from build123d import *

# Parameters (mm, degrees)
SKETCH_1_R      = 23
SKETCH_1_R_2    = 1.75
SKETCH_1_R_3    = 5
EXTRUDE_1_DEPTH = 3
SKETCH_1_3_R    = 5
EXTRUDE_2_DEPTH = 32.75
SKETCH_2_R      = 25
SKETCH_2_R_2    = 1.75
EXTRUDE_3_DEPTH = 3


with BuildPart() as part:
    # 草图1 → 凸台-拉伸1 (new body)
    with BuildSketch(Plane(origin=(0, 0, 0), x_dir=(1, 0, 0), z_dir=(0, 1, 0))):
        with Locations(Location((7.5, 0, 0), (0, 0, 270))):
            Circle(SKETCH_1_R)
        with Locations(Location((27.5, 0, 0), (0, 0, 270))):
            Circle(SKETCH_1_R_2, mode=Mode.SUBTRACT)
        with Locations(Location((-12.5, 0, 0), (0, 0, 270))):
            Circle(SKETCH_1_R_2, mode=Mode.SUBTRACT)
        with Locations(Location((0, 0, 0), (0, 0, 270))):
            Circle(SKETCH_1_R_3, mode=Mode.SUBTRACT)
        with Locations(Location((15, 0, 0), (0, 0, 270))):
            Circle(SKETCH_1_R_3, mode=Mode.SUBTRACT)
    extrude(amount=EXTRUDE_1_DEPTH)

    # 草图1<3> → 凸台-拉伸2 (add)
    with BuildSketch(Plane(origin=(0, 0, 0), x_dir=(1, 0, 0), z_dir=(0, 1, 0))):
        with Locations(Location((0, 0, 0), (0, 0, 270))):
            Circle(SKETCH_1_3_R)
        with Locations(Location((15, 0, 0), (0, 0, 270))):
            Circle(SKETCH_1_3_R)
    extrude(amount=EXTRUDE_2_DEPTH)

    # 草图2 → 凸台-拉伸3 (add)
    with BuildSketch(Plane(origin=(0, 32.75, 0), x_dir=(1, 0, 0), z_dir=(0, 1, 0))):
        with Locations(Location((7.5, 0, 0), (0, 0, 270))):
            Circle(SKETCH_2_R)
        with Locations(Location((-12, 0, 0), (0, 0, 270))):
            Circle(SKETCH_2_R_2, mode=Mode.SUBTRACT)
        with Locations(Location((27, 0, 0), (0, 0, 270))):
            Circle(SKETCH_2_R_2, mode=Mode.SUBTRACT)
    extrude(amount=-EXTRUDE_3_DEPTH)


solid = part.part
Read the model definition and answer for the solid it produces. Units are mm, in the model's axes. A direction names the side the tool comes from. Give positions to 0.01 mm unless a question says otherwise; leave off trailing zeros. Write each loop counter-clockwise with the first axis right and the second up, starting at its lowest first coordinate (ties: lowest second). Pieces come first, ordered by that corner, then holes. Notation, with made-up numbers: (12.25, -9) -> (63.25, -9) arc R16 cw to (63.25, 9) -> close; hole circle Ø1 at (78, 55.5). An arc over 180 degrees is marked (long way). Answer as a JSON object with one key per item and string values. Group by question number.
1) Find section A-A (z = 0). Count the separate pieces of the cut face and the enclosed holes in it, and give its area (3 significant figures).
2) Find section B-B (z = -18). Write down the section's boundary in (x, y), and give its area (3 significant figures).
3) Each of these flat-tipped pins is pushed along its axis until it touches: P1, Ø12, axis at y = 23, z = 16, coming from the -X side; P2, Ø2, axis at x = 4, y = 17.5, coming from the +Z side; P3, Ø3, axis at x = -12.5, z = 0, coming from the -Y side; P4, Ø8, axis at x = 24.5, y = 28, coming from the -Z side. Where does it stop, or does it pass through?
4) The mould has two halves that part along X. Classify faces 4 (the flat face through (8, 32.75, 0)), 5 (the cylindrical face through (28.58, 31.27, 13.44)), 6 (the cylindrical face through (28.735, 31.271, -0.228)): +X half, -X half, draft (parallel to the pull), parting line (faces both ways), or undercut.
5) Consider L1, parallel to X at y = 31, z = 0; L2, parallel to X at y = 1, z = 0; L3, parallel to Y at x = 16, z = -16. Determine where each line is inside the solid, lowest interval first. Write a range as from..to.
6) A tool of negligible diameter and unlimited length cuts with its end or side. For faces 1 (the cylindrical face through (-14.953, 1.479, -4.986)), 2 (the cylindrical face through (-10.265, 31.271, -0.228)), 3 (the cylindrical face through (10.12, 16.19, -1.08)), from which of +Z, -Z, +X, -X, +Y, -Y can it reach the whole face along a straight path? Write none if from no direction.
7) Find section C-C (y = 26.5). Write down the section's boundary in (x, z).
8) Find section D-D (x = 15). Write down the section's boundary in (y, z).
Values follow:
{
 "1": {"separate pieces": "5", "enclosed holes": "1", "area": "781 mm2"},
 "2": {"outline": "(-9.85, 29.75) -> (24.85, 29.75) -> (24.85, 32.75) -> (-9.85, 32.75) -> close; (-6.82, 0) -> (21.82, 0) -> (21.82, 3) -> (-6.82, 3) -> close", "area": "190 mm2"},
 "3": {"P1": "passes through", "P2": "stops at z = 4", "P3": "stops at y = 29.75", "P4": "stops at z = -21.1"},
 "4": {"face 4": "draft", "face 5": "parting line", "face 6": "undercut"},
 "5": {"L1": "x = -17.5..-13.75, -10.25..25.25, 28.75..32.5", "L2": "x = -15.5..-14.25, -10.75..25.75, 29.25..30.5", "L3": "y = 0..3, 29.75..32.75"},
 "6": {"face 1": "-Y", "face 2": "+Y", "face 3": "none"},
 "7": {"outline": "circle Ø10 at (0, 0); circle Ø10 at (15, 0)"},
 "8": {"outline": "(0, -21.74) -> (3, -21.74) -> (3, -5) -> (29.75, -5) -> (29.75, -23.85) -> (32.75, -23.85) -> (32.75, 23.85) -> (29.75, 23.85) -> (29.75, 5) -> (3, 5) -> (3, 21.74) -> (0, 21.74) -> close"}
}
